Geometry: final body of the model. Coordinates: model frame, mm. Face numbers are marked on the shaded views. A direction names the side the tool comes from. Give positions to 0.01 mm unless a question says otherwise; leave off trailing zeros. Write each loop counter-clockwise with the first axis right and the second up, starting at its lowest first coordinate (ties: lowest second). Pieces come first, ordered by that corner, then holes.
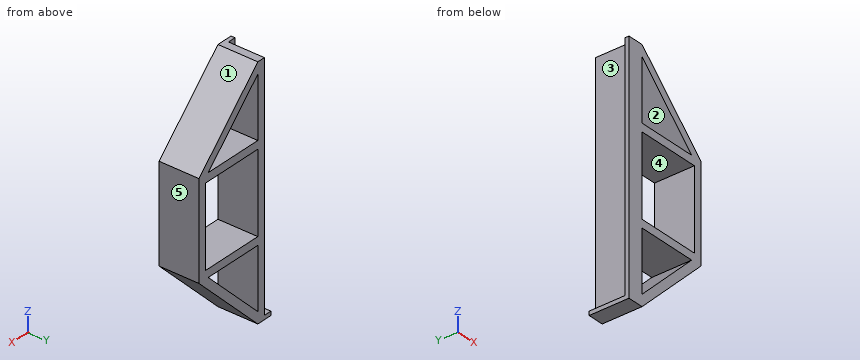
Autodesk Inventor part; units mm, degrees
ref_plane "YZ Plane" through (0, 0, 0) normal (1, 0, 0) x (0, 1, 0)
ref_plane "XZ Plane" through (0, 0, 0) normal (0, 1, 0) x (-1, 0, 0)
ref_plane "XY Plane" through (0, 0, 0) normal (0, 0, 1) x (1, 0, 0)
sketch "Sketch1" plane through (0, 0, 0) normal (0, 1, 0) x (-1, 0, 0)
  line L0 (9, 10) -> (-7, 10)
  line L1 (-7, 10) -> (-7, -10)
  line L2 (-7, -10) -> (9, -10)
  line L3 (9, -10) -> (9, 10)
  line L4 (9, 10) -> (-7, -10) construction
  line L5 (-7, 10) -> (9, -10) construction
  line L6 (-9, 12) -> (11, 12)
  line L7 (11, 12) -> (11, -12)
  line L8 (11, -12) -> (-9, -12)
  line L9 (-9, -12) -> (-9, 12)
  line L10 (-9, 12) -> (9, 30)
  line L11 (-9, 12) -> (21.2472, 12) construction
  line L12 (11, 12) -> (11, 30)
  line L13 (-9, -12) -> (9, -30)
  line L14 (-9, -12) -> (29.5291, -12) construction
  line L15 (11, -12) -> (11, -30)
  line L16 (9, 12) -> (9, 29.1716)
  line L17 (-6.1716, -12) -> (9, -27.1716)
  line L18 (9, -27.1716) -> (9, -12)
  line L19 (11, 12) -> (11, 10)
  line L20 (11, 12) -> (9, 12)
  line L21 (-8.1716, 12) -> (-9, 12)
  line L22 (-9, -12) -> (-6.1716, -12)
  line L23 (11, -12) -> (9, -12)
  line L24 (9, 29.1716) -> (9, 30)
  line L25 (9, 30) -> (11, 30)
  line L26 (9, -27.1716) -> (11, -27.1716)
  line L27 (9, -27.1716) -> (9, -30)
  line L28 (9, -30) -> (11, -30)
  line L29 (11, 12) -> (9, 12)
  line L30 (-8.1716, 12) -> (-9, 12)
  line L31 (-6.1716, -12) -> (9, -12)
  line L32 (11, -12) -> (9, -12)
  line L33 (9, 30) -> (9, 28)
  line L34 (9, 27.1716) -> (-6.1716, 12)
  line L35 (9, 27.1716) -> (9, 30)
  line L36 (9, 27.1716) -> (-6.1716, 12)
  line L37 (-9, 12) -> (-6.1716, 12)
  line L38 (9, 30) -> (-9, 12)
  point P0 (0, 0)
  point P1 (1, 0)
  dimension "d0" = 16
  dimension "d1" = 20
  dimension "d2" = 2
  dimension "d3" = 45
  dimension "d4" = 45
  dimension "d5" = 2
  dimension "d6" = 2
  dimension "d12" = 2
extrude "Extrusion2" add sketch "Sketch1" along normal blind 10 contours L10 L24 L16 L34 L6 | L6 L7 L8 L9 | L8 L17 L27 L13 | L25 L12 L6 L16 L24 | L27 L26 L15 L28 | L8 L15 L26 L18
sketch "Sketch3" plane through (0, 0, 0) normal (0, -1, 0) x (1, 0, 0)
  line L0 (-11, 30) -> (-13, 30)
  line L1 (-13, 30) -> (-13, -30)
  line L2 (-13, -30) -> (-11, -30)
  line L3 (-11, -30) -> (-11, 30)
  line L4 (-11, -30) -> (-11, 30)
  point P0 (0, 0)
  dimension "d15" = 2
  dimension "d16" = 60
extrude "Extrusion3" add sketch "Sketch3" against normal blind 1
sketch "Sketch4" plane through (-9, 10, -30) normal (0, 0, -1) x (-1, 0, 0)
  line L0 (2, -9) -> (2, 0)
  line L1 (2, 0) -> (2, -9)
  line L2 (4, -9) -> (2, -9)
  line L3 (2, -9) -> (4, -9)
  line L4 (4, -9) -> (4, 0)
  line L5 (4, 0) -> (2, 0)
  point P0 (-9, -10)
extrude "Extrusion4" add sketch "Sketch4" against normal blind 1
properties part number "Motor_Org"
Item 1: Line query: L1, parallel to X at y = 7.5, z = 7; L2, parallel to Z at x = -0.5, y = 3.25; L3, parallel to Z at x = -8.5, y = 7.25. Output: solid intervals per line, ascending.
Found:
L1: x = -11 to -9, 7 to 9
L2: z = -21.5 to -18.67, -12 to -10, 10 to 12, 18.67 to 21.5
L3: z = -29.5 to -26.67, -12 to -10, 10 to 12, 26.67 to 29.5
Item 2: Section A-A, the plane z = 0.5. Return the cut outline in (x, y), plus the area to 3 significant figures.
Found:
outline: (-13, 0) - (-9, 0) - (-9, 10) - (-11, 10) - (-11, 1) - (-13, 1) - close; (7, 0) - (9, 0) - (9, 10) - (7, 10) - close
area: 42.0 mm2
Item 3: Reachability of the marked faces 4 and 5 from +Z, -Z, +X, -X, +Y, -Y: full face, straight path, thin tool, end or side. Return the list, or none.
Found:
face 4: +Y, -Y
face 5: +Z, -Z, +X, +Y, -Y
Item 4: Section B-B, the plane y = 9.25. Return the cut outline in (x, z).
Found:
outline: (-13, -30) - (-9, -30) - (9, -12) - (9, 12) - (-9, 30) - (-11, 30) - (-11, -29) - (-13, -29) - close; hole (-9, -27.17) - (6.17, -12) - (-9, -12) - close; hole (-9, -10) - (7, -10) - (7, 10) - (-9, 10) - close; hole (-9, 12) - (6.17, 12) - (-9, 27.17) - close
Item 5: Pin query (flat end, axial travel): pin 1 Ø3 at (x, y) = (3, 4.5) entering from -Z; pin 2 Ø4.5 at (y, z) = (3.5, 4.5) entering from -X; pin 3 Ø1 at (x, z) = (-12.5, 6.5) entering from +Y; pin 4 Ø12 at (x, z) = (5.5, -1) entering from +Y. Return the tip coordinate at first contact, or that it passes through.
Found:
pin 1: stops at z = -19.5
pin 2: stops at x = -11
pin 3: stops at y = 1
pin 4: stops at y = 10
Item 6: Section C-C, the plane x = 0.75. Return the cut outline in (y, z).
Found:
outline: (0, -20.25) - (10, -20.25) - (10, -17.42) - (0, -17.42) - close; (0, -12) - (10, -12) - (10, -10) - (0, -10) - close; (0, 10) - (10, 10) - (10, 12) - (0, 12) - close; (0, 17.42) - (10, 17.42) - (10, 20.25) - (0, 20.25) - close
Item 7: Pull-direction query (X, two-part tool) for the marked faces 1, 2 and 3; classes: +X half, -X half, draft (parallel to the pull), parting line (faces both ways), or undercut.
Found:
face 1: +X half
face 2: undercut
face 3: -X half
Item 8: Section D-D, the plane z = -11. Return the cut outline in (x, y), plus the area to 3 significant figures.
Found:
outline: (-13, 0) - (9, 0) - (9, 10) - (-11, 10) - (-11, 1) - (-13, 1) - close
area: 202 mm2
